from build123d import *

# Parameters (mm, degrees)
SKETCH1_R           = 4.765
SKETCH1_R_2         = 1.59
BOSS_EXTRUDE1_DEPTH = 9.5
CHAMFER1_SIZE       = 2.54
CHAMFER1_SIZE_2     = 7.62
CHAMFER2_SIZE       = 7.62
CHAMFER2_SIZE_2     = 2.54
SKETCH2_W           = 9.53
SKETCH2_H           = 9.53
CUT_EXTRUDE1_DEPTH  = 56.26045331
CUT_EXTRUDE2_DEPTH  = 56.26045331


with BuildPart() as part:
    # Sketch1 → Boss-Extrude1 (new, symmetric)
    with BuildSketch(Plane.XY):
        with BuildLine():
            Line((0, 0), (0, -5))
            Line((0, -5), (12.518490754, -10.837468107))
            ThreePointArc((12.518490754, -10.837468107), (15.709887401, -17.046058803), (22.23, -19.54))
            Line((22.23, -19.54), (50.81, -14.77))
            Line((50.81, -14.77), (50.81, -9.77))
            Line((50.81, -9.77), (32, -9.77))
            ThreePointArc((32, -9.77), (29.138433252, -2.861566748), (22.23, 0))
            Line((22.23, 0), (0, 0))
        make_face()
        with Locations((22.23, -9.77)):
            Circle(SKETCH1_R, mode=Mode.SUBTRACT)
        with Locations((2.54, -2.54)):
            Circle(SKETCH1_R_2, mode=Mode.SUBTRACT)
        with Locations((48.27, -12.31)):
            Circle(SKETCH1_R_2, mode=Mode.SUBTRACT)
    extrude(amount=BOSS_EXTRUDE1_DEPTH, both=True)

    # Chamfer1
    # the kernel refuses this chamfer: 7.62, 2.54 mm, written as the material it takes off along each edge
    with BuildSketch(Plane(origin=(0, 19.774364901, -9.5), x_dir=(-0.10902612017980703, 0, 0.9940388851139267), z_dir=(0, -1, 0))) as chamfer1_piece_1:
        Polygon((CHAMFER1_SIZE * 0.994038885114, -CHAMFER1_SIZE * 0.10902612018), (-CHAMFER1_SIZE_2 * 0.10902612018, -CHAMFER1_SIZE_2 * 0.994038885114), (0, 0), align=None)
    extrude(amount=44.548729802, mode=Mode.SUBTRACT)
    with BuildSketch(Plane(origin=(0, 19.774364901, 9.5), x_dir=(-0.10902612017980703, 0, -0.9940388851139267), z_dir=(0, -1, 0)), Plane(origin=(50.81, -34.544364901, 9.5), x_dir=(0.10902612017980588, 0, -0.9940388851139268), z_dir=(0, 1, 0))) as chamfer1_piece_2:
        Polygon((CHAMFER1_SIZE * 0.994038885114, CHAMFER1_SIZE * 0.10902612018), (-CHAMFER1_SIZE_2 * 0.10902612018, CHAMFER1_SIZE_2 * 0.994038885114), (0, 0), align=None)
    extrude(amount=44.548729802, mode=Mode.SUBTRACT)

    # Chamfer2
    # the kernel refuses this chamfer: 7.62, 2.54 mm, written as the material it takes off along each edge
    with BuildSketch(Plane(origin=(50.81, -34.544364901, -9.5), x_dir=(-0.9999257509361694, 0, -0.01218575458219919), z_dir=(0, 1, 0))) as chamfer2_piece_1:
        Polygon((CHAMFER2_SIZE * 0.999925750936, CHAMFER2_SIZE * 0.0121857545822), (-CHAMFER2_SIZE_2 * 0.0121857545822, CHAMFER2_SIZE_2 * 0.999925750936), (0, 0), align=None)
    extrude(amount=44.548729802, mode=Mode.SUBTRACT)

    # Sketch2 → Cut-Extrude1 (cut, through all)
    with BuildSketch(Plane(origin=(0, 0, 0), x_dir=(1, 0, 0), z_dir=(0, 1, 0))):
        with Locations((4.765, 0)):
            Rectangle(SKETCH2_W, SKETCH2_H)
        with Locations((46.045, 0)):
            Rectangle(SKETCH2_W, SKETCH2_H)
    extrude(amount=-CUT_EXTRUDE1_DEPTH, mode=Mode.SUBTRACT)

    # Sketch3 → Cut-Extrude2 (cut, through all)
    with BuildSketch(Plane(origin=(0, 0, 0), x_dir=(1, 0, 0), z_dir=(0, 1, 0))):
        with BuildLine():
            Line((18.42, 5.08), (28.58, 5.08))
            ThreePointArc((28.58, 5.08), (33.66, 0), (28.58, -5.08))
            Line((28.58, -5.08), (18.42, -5.08))
            ThreePointArc((18.42, -5.08), (13.34, 0), (18.42, 5.08))
        make_face()
    extrude(amount=-CUT_EXTRUDE2_DEPTH, mode=Mode.SUBTRACT)


solid = part.part
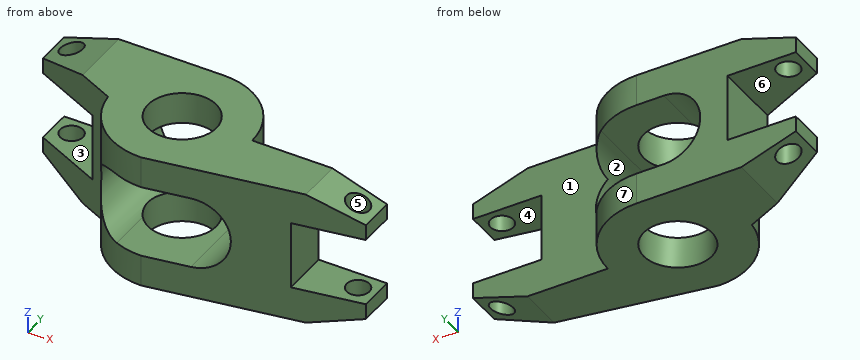
Part model, mm, in its own coordinate system. Face numbers are marked on the shaded views. A direction names the side the tool comes from. Give positions to 0.01 mm unless a question says otherwise; leave off trailing zeros. Order: outer loops, then holes, each group sorted by start corner. A loop starts at its lowest first (then second) coordinate and runs counter-clockwise, first axis right, second up. Notation, with made-up numbers: (10.25, 81) - (14.25, 81) arc R5 ccw to (14.25, 86) - close; hole circle Ø1 at (66.25, -0.75). An arc over 180 degrees is marked (long way). One line per question, with ' | ' between items.
1. Drop flat-ended pins along their axis: P1, Ø4, axis at x = 48.27, y = -12.31, coming from the -Z side; P2, Ø1.9, axis at x = 2.54, y = -2.54, coming from the +Z side; P3, Ø3.5, axis at x = 47, y = -14.5, coming from the -Z side; P4, Ø1.5, axis at x = 6, y = -5, coming from the -Z side. Give the stop position or say it passes through.
Filled in:
P1: z = -8.47 | P2: through | P3: z = -8.81 | P4: z = -9.21
2. Band-saw the part on D-D on y = -18. List the corners of the cut face in (x, z), then the cut area to 3 significant figures.
Filled in:
outline: (16.97, -9.5) - (31.46, -9.5) - (31.46, -4.19) arc R5.08 cw to (28.58, -5.08) - (18.42, -5.08) arc R5.08 cw to (16.97, -4.87) - close; (16.97, 4.87) arc R5.08 cw to (18.42, 5.08) - (28.58, 5.08) arc R5.08 cw to (31.46, 4.19) - (31.46, 9.5) - (16.97, 9.5) - close | area: 130 mm²
3. Pull direction X, two halves, no side cores. Call the marked faces 5, 6 and 7: +X half, -X half, draft (parallel to the pull), parting line (faces both ways), or undercut.
Filled in:
face 5: undercut | face 6: draft | face 7: +X half
4. Band-saw the part on C-C on x = 6. List the corners of the cut face in (y, z) (3 decimals).
Filled in:
outline: (-7.798, -8.96) - (0, -8.96) - (0, -4.765) - (-7.798, -4.765) - close; (-7.798, 4.765) - (0, 4.765) - (0, 8.96) - (-7.798, 8.96) - close
5. Band-saw the part on B-B on x = 21.5. List the corners of the cut face in (y, z), then the cut area to 3 significant figures.
Filled in:
outline: (-19.51, -9.5) - (-14.48, -9.5) - (-14.48, -5.08) - (-19.51, -5.08) - close; (-19.51, 5.08) - (-14.48, 5.08) - (-14.48, 9.5) - (-19.51, 9.5) - close; (-5.06, -9.5) - (0, -9.5) - (0, -5.08) - (-5.06, -5.08) - close; (-5.06, 5.08) - (0, 5.08) - (0, 9.5) - (-5.06, 9.5) - close | area: 89.2 mm²
6. Drill centre lines: probe 1 along Y at (x, z) = (48.27, 5.95); probe 2 along Y at (x, z) = (3, -6.25); probe 3 along X at (y, z) = (-12.31, 6.6). Where is each one in solid material? Low to high.
Filled in:
probe 1: -15.19 to -13.9, -10.72 to -9.77 | probe 2: -6.4 to -4.06, -1.02 to 0 | probe 3: 12.8 to 18.2, 26.26 to 46.68, 49.86 to 50.81
7. Which spindle directions (+Z, -Z, +X, -X, +Y, -Y) get a long thin tool onto all of the face, cutting with end or side? Do the marked faces 1, 2, 3 and 4. Say none if no direction does.
Filled in:
face 1: +Z, -Z, +X, +Y | face 2: +Y, -Y | face 3: -X, +Y, -Y | face 4: +X, +Y, -Y
8. Band-saw the part on A-A on z = 0. List the corners of the cut face in (x, y).
Filled in:
outline: (9.53, -9.44) - (12.52, -10.84) arc R9.77 ccw to (13.34, -13.82) - (13.34, 0) - (9.53, 0) - close; (33.66, -17.63) - (41.28, -16.36) - (41.28, -9.77) - (33.66, -9.77) - close
